from build123d import *

# Parameters (mm, degrees)
F0_R     = 1.27
F0_R_2   = 1.5875
F1_DEPTH = 2.54


with BuildPart() as f1:
    # F0 (on Front) → F1 (new body)
    with BuildSketch(Plane.XZ):
        with BuildLine():
            Line((106.68, 41.302181), (-106.680917, 41.302181))
            ThreePointArc((-106.680917, 41.302181), (-107.578942, 40.930207), (-107.950917, 40.032181))
            Line((-107.950917, 40.032181), (-107.950917, -40.005))
            ThreePointArc((-107.950917, -40.005), (-107.578942, -40.903026), (-106.680917, -41.275))
            Line((-106.680917, -41.275), (106.68, -41.275))
            ThreePointArc((106.68, -41.275), (107.578026, -40.903026), (107.95, -40.005))
            Line((107.95, -40.005), (107.95, 40.032181))
            ThreePointArc((107.95, 40.032181), (107.578026, 40.930207), (106.68, 41.302181))
        make_face()
        with Locations((-104.775917, -38.1)):
            Circle(F0_R, mode=Mode.SUBTRACT)
        with Locations((-75.692, -33.2105)):
            Circle(F0_R_2, mode=Mode.SUBTRACT)
        with Locations((-47.752, -33.2105)):
            Circle(F0_R_2, mode=Mode.SUBTRACT)
        with Locations((-19.812, -33.2105)):
            Circle(F0_R_2, mode=Mode.SUBTRACT)
        with BuildLine():
            ThreePointArc((-77.47, -10.406757), (-83.82, -30.63875), (-90.17, -10.406757))
            Line((-90.17, -10.406757), (-90.17, -8.817245))
            ThreePointArc((-90.17, -8.817245), (-83.82, -7.076138), (-77.47, -8.817245))
            Line((-77.47, -8.817245), (-77.47, -10.406757))
        make_face(mode=Mode.SUBTRACT)
        with BuildLine():
            ThreePointArc((-49.53, -10.406757), (-55.88, -30.63875), (-62.23, -10.406757))
            Line((-62.23, -10.406757), (-62.23, -8.817245))
            ThreePointArc((-62.23, -8.817245), (-55.88, -7.076138), (-49.53, -8.817245))
            Line((-49.53, -8.817245), (-49.53, -10.406757))
        make_face(mode=Mode.SUBTRACT)
        with Locations((-91.948, -5.842)):
            Circle(F0_R_2, mode=Mode.SUBTRACT)
        with Locations((-64.008, -5.842)):
            Circle(F0_R_2, mode=Mode.SUBTRACT)
        with BuildLine():
            ThreePointArc((-21.59, -10.406757), (-27.94, -30.63875), (-34.29, -10.406757))
            Line((-34.29, -10.406757), (-34.29, -8.817245))
            ThreePointArc((-34.29, -8.817245), (-27.94, -7.076138), (-21.59, -8.817245))
            Line((-21.59, -8.817245), (-21.59, -10.406757))
        make_face(mode=Mode.SUBTRACT)
        with Locations((-36.068, -5.842)):
            Circle(F0_R_2, mode=Mode.SUBTRACT)
        with Locations((-8.128, -5.842)):
            Circle(F0_R_2, mode=Mode.SUBTRACT)
        with Locations((8.128, -33.2105)):
            Circle(F0_R_2, mode=Mode.SUBTRACT)
        with Locations((36.068, -33.2105)):
            Circle(F0_R_2, mode=Mode.SUBTRACT)
        with Locations((104.775, -38.1)):
            Circle(F0_R, mode=Mode.SUBTRACT)
        with BuildLine():
            ThreePointArc((6.35, -10.406757), (0, -30.63875), (-6.35, -10.406757))
            Line((-6.35, -10.406757), (-6.35, -8.817245))
            ThreePointArc((-6.35, -8.817245), (0, -7.076138), (6.35, -8.817245))
            Line((6.35, -8.817245), (6.35, -10.406757))
        make_face(mode=Mode.SUBTRACT)
        with BuildLine():
            ThreePointArc((34.29, -10.406757), (27.94, -30.63875), (21.59, -10.406757))
            Line((21.59, -10.406757), (21.59, -8.817245))
            ThreePointArc((21.59, -8.817245), (27.94, -7.076138), (34.29, -8.817245))
            Line((34.29, -8.817245), (34.29, -10.406757))
        make_face(mode=Mode.SUBTRACT)
        with Locations((19.812, -5.842)):
            Circle(F0_R_2, mode=Mode.SUBTRACT)
        with Locations((-75.692, 5.842)):
            Circle(F0_R_2, mode=Mode.SUBTRACT)
        with BuildLine():
            ThreePointArc((-77.47, 28.645743), (-83.82, 8.41375), (-90.17, 28.645743))
            Line((-90.17, 28.645743), (-90.17, 30.235255))
            ThreePointArc((-90.17, 30.235255), (-83.82, 31.976362), (-77.47, 30.235255))
            Line((-77.47, 30.235255), (-77.47, 28.645743))
        make_face(mode=Mode.SUBTRACT)
        with BuildLine():
            ThreePointArc((-49.53, 28.645743), (-55.88, 8.41375), (-62.23, 28.645743))
            Line((-62.23, 28.645743), (-62.23, 30.235255))
            ThreePointArc((-62.23, 30.235255), (-55.88, 31.976362), (-49.53, 30.235255))
            Line((-49.53, 30.235255), (-49.53, 28.645743))
        make_face(mode=Mode.SUBTRACT)
        with Locations((-47.752, 5.842)):
            Circle(F0_R_2, mode=Mode.SUBTRACT)
        with Locations((-19.812, 5.842)):
            Circle(F0_R_2, mode=Mode.SUBTRACT)
        with BuildLine():
            ThreePointArc((-21.59, 28.645743), (-27.94, 8.41375), (-34.29, 28.645743))
            Line((-34.29, 28.645743), (-34.29, 30.235255))
            ThreePointArc((-34.29, 30.235255), (-27.94, 31.976362), (-21.59, 30.235255))
            Line((-21.59, 30.235255), (-21.59, 28.645743))
        make_face(mode=Mode.SUBTRACT)
        with Locations((-91.948, 33.2105)):
            Circle(F0_R_2, mode=Mode.SUBTRACT)
        with Locations((-104.775917, 38.127181)):
            Circle(F0_R_2, mode=Mode.SUBTRACT)
        with Locations((-64.008, 33.2105)):
            Circle(F0_R_2, mode=Mode.SUBTRACT)
        with Locations((-36.068, 33.2105)):
            Circle(F0_R_2, mode=Mode.SUBTRACT)
        with Locations((-8.128, 33.2105)):
            Circle(F0_R_2, mode=Mode.SUBTRACT)
        with Locations((8.128, 5.842)):
            Circle(F0_R_2, mode=Mode.SUBTRACT)
        with Locations((36.068, 5.842)):
            Circle(F0_R_2, mode=Mode.SUBTRACT)
        with BuildLine():
            ThreePointArc((6.35, 28.645743), (0, 8.41375), (-6.35, 28.645743))
            Line((-6.35, 28.645743), (-6.35, 30.235255))
            ThreePointArc((-6.35, 30.235255), (0, 31.976362), (6.35, 30.235255))
            Line((6.35, 30.235255), (6.35, 28.645743))
        make_face(mode=Mode.SUBTRACT)
        with BuildLine():
            ThreePointArc((34.29, 28.645743), (27.94, 8.41375), (21.59, 28.645743))
            Line((21.59, 28.645743), (21.59, 30.235255))
            ThreePointArc((21.59, 30.235255), (27.94, 31.976362), (34.29, 30.235255))
            Line((34.29, 30.235255), (34.29, 28.645743))
        make_face(mode=Mode.SUBTRACT)
        with Locations((19.812, 33.2105)):
            Circle(F0_R_2, mode=Mode.SUBTRACT)
        with Locations((104.775, 38.127181)):
            Circle(F0_R, mode=Mode.SUBTRACT)
    extrude(amount=F1_DEPTH)


solid = f1.part
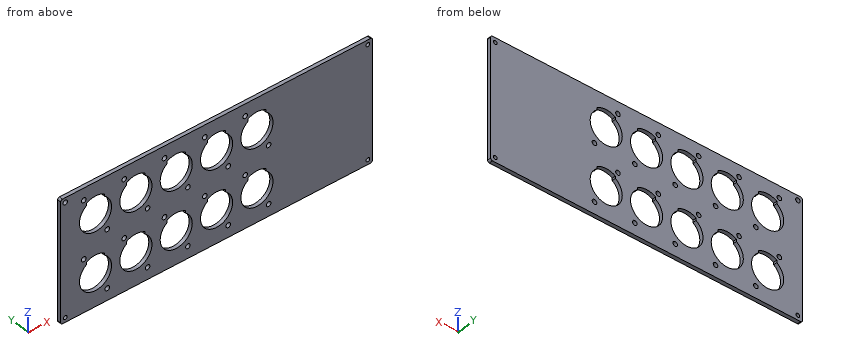
The listing builds one solid part. Answer for the finished solid, in the listing's coordinates (mm). Give positions to 0.01 mm unless a question says otherwise; leave off trailing zeros. Write each loop counter-clockwise with the first axis right and the second up, starting at its lowest first coordinate (ties: lowest second). Pieces come first, ordered by that corner, then holes.
1) Section B-B (z = 14.5) is taken. Write down the section's boundary in (x, y), and give its area (3 significant figures).
2) Section A-A (x = -83.82) is taken. Write down the section's boundary in (y, z) (3 decimals), and give its area (3 significant figures).
3) Section C-C (y = -0.6) is taken. Count the separate pieces of the cut face and the enclosed holes in it, and give its area (3 significant figures).
4) Find the intervals of material crossed by L1, parallel to X at y = -2.1, z = 19.5; L2, parallel to Z at x = 0.5, y = -0.6 (1 decimal); L3, parallel to X at y = -0.6, z = -6, in increasing order.
Response:
1. outline: (-107.95, -2.54) - (-93.73, -2.54) - (-93.73, 0) - (-107.95, 0) - close; (-73.91, -2.54) - (-65.79, -2.54) - (-65.79, 0) - (-73.91, 0) - close; (-45.97, -2.54) - (-37.85, -2.54) - (-37.85, 0) - (-45.97, 0) - close; (-18.03, -2.54) - (-9.91, -2.54) - (-9.91, 0) - (-18.03, 0) - close; (9.91, -2.54) - (18.03, -2.54) - (18.03, 0) - (9.91, 0) - close; (37.85, -2.54) - (107.95, -2.54) - (107.95, 0) - (37.85, 0) - close
1. area: 297 mm2
2. outline: (-2.54, -41.275) - (0, -41.275) - (0, -30.639) - (-2.54, -30.639) - close; (-2.54, -7.076) - (0, -7.076) - (0, 8.414) - (-2.54, 8.414) - close; (-2.54, 31.976) - (0, 31.976) - (0, 41.302) - (-2.54, 41.302) - close
2. area: 90.0 mm2
3. separate pieces: 1
3. enclosed holes: 34
3. area: 13,600 mm2
4. L1: x = -107.95 to -94.93, -72.71 to -66.99, -44.77 to -39.05, -16.83 to -11.11, 11.11 to 16.83, 39.05 to 107.95
4. L2: z = -41.3 to -30.6, -7.1 to 8.4, 32 to 41.3
4. L3: x = -107.95 to -93.53, -90.37 to -65.59, -62.43 to -37.65, -34.49 to -9.71, -6.55 to 18.23, 21.39 to 107.95
